from build123d import *

# Parameters (mm, degrees)
SKETCH1_W           = 226
SKETCH1_H           = 84
BOSS_EXTRUDE1_DEPTH = 20
BOSS_EXTRUDE2_DEPTH = 20
SKETCH4_W           = 1.65
SKETCH4_H           = 46.5
BOSS_EXTRUDE3_DEPTH = 5
SKETCH4_2_W         = 1.65
SKETCH4_2_H         = 46.5
CUT_EXTRUDE1_DEPTH  = 5
CAVITY2_START       = 416.690531323
CAVITY2_DEPTH       = 123.991681054
CAVITY2_START_2     = 387.890531323
CAVITY2_2_DEPTH     = 14.5
CAVITY2_3_DEPTH     = 3.8
CAVITY2_4_DEPTH     = 26
CAVITY2_START_3     = 542.682212377
CAVITY2_5_DEPTH     = 12.45
CAVITY2_6_OUTLINE_W = 10.967659298
CAVITY2_6_OUTLINE_H = 10.05
CAVITY2_6_DEPTH     = 1.2
CAVITY2_START_4     = 553.932212377
CAVITY2_7_OUTLINE_W = 10.967659298
CAVITY2_7_OUTLINE_H = 10.05
CAVITY2_7_DEPTH     = 1.2
SKETCH7_W           = 10.05
SKETCH7_H           = 10.05
CUT_EXTRUDE2_DEPTH  = 12


# Read off the part's stored shape, not the designer's step: Cavity2
with BuildPart() as part:
    # Sketch1 → Boss-Extrude1 (new body)
    with BuildSketch(Plane(origin=(375.872687737, 0, 1298.443562055), x_dir=(1, 0, 0), z_dir=(0, 1, 0))):
        with Locations((113, -81.370523073)):
            Rectangle(SKETCH1_W, SKETCH1_H)
    extrude(amount=BOSS_EXTRUDE1_DEPTH)

    # Sketch2 → Boss-Extrude2 (add)
    with BuildSketch(Plane.XZ):
        Polygon((601.872687737, 1377.314085128), (601.872687737, 1382.314085128), (611.872687737, 1389.814085128), (611.872687737, 1369.814085128), align=None)
    extrude(amount=-BOSS_EXTRUDE2_DEPTH)

    # Sketch4 → Boss-Extrude3 (add)
    with BuildSketch(Plane(origin=(0, 20, 0), x_dir=(1, 0, 0), z_dir=(0, 1, 0))):
        with Locations((573.047687737, -1379.814085128)):
            Rectangle(SKETCH4_W, SKETCH4_H)
    extrude(amount=-BOSS_EXTRUDE3_DEPTH)

    # Sketch4<2> → Cut-Extrude1 (cut)
    with BuildSketch(Plane(origin=(0, 20, 0), x_dir=(1, 0, 0), z_dir=(0, 1, 0))):
        with Locations((573.047687737, -1379.814085128)):
            Rectangle(SKETCH4_2_W, SKETCH4_2_H)
    extrude(amount=-CUT_EXTRUDE1_DEPTH, mode=Mode.SUBTRACT)

    # Cavity2 outline → Cavity2 (cut)
    with BuildSketch(Plane.YZ.offset(CAVITY2_START)):
        with BuildLine():
            ThreePointArc((20, 1387.257061845), (17.532340702, 1379.800377592), (20, 1372.34369334))
            Line((20, 1372.34369334), (20, 1387.257061845))
        make_face()
    extrude(amount=CAVITY2_DEPTH, mode=Mode.SUBTRACT)

    # Cavity2 2 outline → Cavity2 2 (cut)
    with BuildSketch(Plane.YZ.offset(CAVITY2_START_2)):
        with BuildLine():
            ThreePointArc((20, 1394.13921088), (12.532340702, 1379.800377593), (20, 1365.461544305))
            Line((20, 1365.461544305), (20, 1394.13921088))
        make_face()
    extrude(amount=CAVITY2_2_DEPTH, mode=Mode.SUBTRACT)

    # Cavity2 3 outline → Cavity2 3 (cut)
    with BuildSketch(Plane.YZ.offset(CAVITY2_START_2)):
        with BuildLine():
            Line((20, 1394.13921088), (20, 1399.050377582))
            Line((20, 1399.050377582), (10.782340682, 1399.050377573))
            Line((10.782340682, 1399.050377573), (10.782340722, 1360.550377573))
            Line((10.782340722, 1360.550377573), (20, 1360.550377582))
            Line((20, 1360.550377582), (20, 1365.461544305))
            ThreePointArc((20, 1365.461544305), (12.532340702, 1379.800377593), (20, 1394.13921088))
        make_face()
    extrude(amount=CAVITY2_3_DEPTH, mode=Mode.SUBTRACT)

    # Cavity2 4 outline → Cavity2 4 (cut)
    with BuildSketch(Plane.YZ.offset(CAVITY2_START)):
        with BuildLine():
            Line((20, 1387.257061845), (20, 1389.636771243))
            ThreePointArc((20, 1389.636771243), (15.982340702, 1379.800377593), (20, 1369.963983943))
            Line((20, 1369.963983943), (20, 1372.34369334))
            ThreePointArc((20, 1372.34369334), (17.532340702, 1379.800377592), (20, 1387.257061845))
        make_face()
    extrude(amount=CAVITY2_4_DEPTH, mode=Mode.SUBTRACT)

    # Cavity2 5 outline → Cavity2 5 (cut)
    with BuildSketch(Plane.YZ.offset(CAVITY2_START_3)):
        Polygon((20, 1386.025377593), (7.832340702, 1386.025377593), (7.832340702, 1373.575377593), (20, 1373.575377593), (20, 1374.775377593), (9.032340702, 1374.775377593), (9.032340702, 1384.825377593), (20, 1384.825377593), align=None)
    extrude(amount=CAVITY2_5_DEPTH, mode=Mode.SUBTRACT)

    # Cavity2 6 outline → Cavity2 6 (cut)
    with BuildSketch(Plane.YZ.offset(CAVITY2_START_3)):
        with Locations((14.516170351, 1379.800377593)):
            Rectangle(CAVITY2_6_OUTLINE_W, CAVITY2_6_OUTLINE_H)
    extrude(amount=CAVITY2_6_DEPTH, mode=Mode.SUBTRACT)

    # Cavity2 7 outline → Cavity2 7 (cut)
    with BuildSketch(Plane.YZ.offset(CAVITY2_START_4)):
        with Locations((14.516170351, 1379.800377593)):
            Rectangle(CAVITY2_7_OUTLINE_W, CAVITY2_7_OUTLINE_H)
    extrude(amount=CAVITY2_7_DEPTH, mode=Mode.SUBTRACT)

    # Sketch7 → Cut-Extrude2 (cut)
    with BuildSketch(Plane(origin=(0, 20, 0), x_dir=(1, 0, 0), z_dir=(0, 1, 0))):
        with Locations((548.907212377, -1379.800377593)):
            Rectangle(SKETCH7_W, SKETCH7_H)
    extrude(amount=-CUT_EXTRUDE2_DEPTH, mode=Mode.SUBTRACT)


solid = part.part
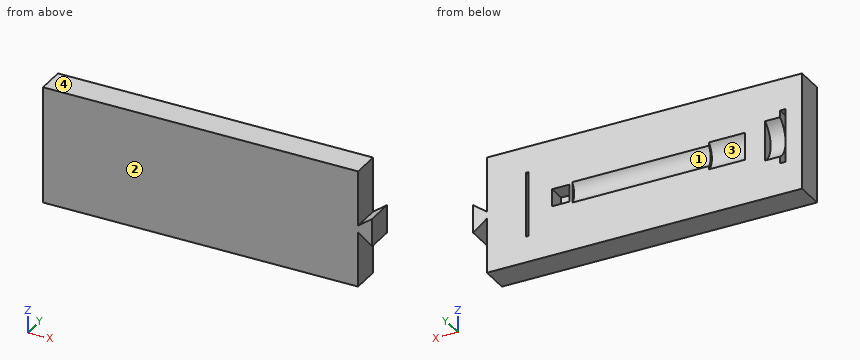
Design review of the part built by this model. Coordinates are the model's own, in mm. Face numbers are marked on the shaded views. A direction names the side the tool comes from. Coordinates: 2 decimals unless noted, no trailing zeros. Loops run counter-clockwise (first coordinate to the right, second up) from the corner with the lowest first, then second, coordinate; pieces in that order, holes last.
Item 1: Clearance check with flat-ended pins moving along their axes: pin 1 (5 mm diameter, centred on x = 451, z = 1379.5, fed in from -Y); pin 2 (1.9 mm diameter, centred on x = 389, z = 1376, fed in from +Y); pin 3 (6 mm diameter, centred on y = 5.5, z = 1395, fed in from +X). State where each tip first meets the part, or that it passes through.
Completed:
pin 1: stops at y = 0
pin 2: stops at y = 10.78
pin 3: stops at x = 601.87
Item 2: Add section A-A (y = 2.5). Write out the cut boundary in (x, z).
Completed:
outline: (375.87, 1337.81) - (601.87, 1337.81) - (601.87, 1377.31) - (611.87, 1369.81) - (611.87, 1389.81) - (601.87, 1382.31) - (601.87, 1421.81) - (375.87, 1421.81) - close
Item 3: Wall thickness on L1, parallel to X at y = 17.75, z = 1368; L2, parallel to X at y = 13.25, z = 1387; L3, parallel to X at y = 5.75, z = 1411.5: over which ranges is each line inside the solid? List them lowest first.
Completed:
L1: x = 375.87 to 387.89, 402.39 to 572.22, 573.87 to 601.87
L2: x = 375.87 to 387.89, 391.69 to 601.87, 608.12 to 611.87
L3: x = 375.87 to 601.87
Item 4: Add section C-C (z = 1406.5). Write out the cut boundary in (x, y).
Completed:
outline: (375.87, 0) - (601.87, 0) - (601.87, 20) - (375.87, 20) - close
Item 5: Draft analysis for pull direction X (two halves, no side actions). For the marked faces 3 and 4, state which applies: pulls with the +X half, pulls with the -X half, needs draft (parallel to the pull), parting line crosses it, or undercut.
Completed:
face 3: undercut
face 4: needs draft
Item 6: Add section B-B (x = 546). Write out the cut boundary in (y, z), and give its area (3 significant figures).
Completed:
outline: (0, 1337.81) - (20, 1337.81) - (20, 1373.58) - (7.83, 1373.58) - (7.83, 1386.03) - (20, 1386.03) - (20, 1421.81) - (0, 1421.81) - close
area: 1,530 mm2
Item 7: For the marked faces 1 and 2, list the 3-axis set-ups (+Z, -Z, +X, -X, +Y, -Y) from which the entire face can be reached by the end or side of a thin tool; tool diameter is ignored.
Completed:
face 1: +Y
face 2: +Z, -Z, +X, -X, -Y
